Geometry: final body of the model. Coordinates: model frame, mm. A direction names the side the tool comes from. Coordinates: 2 decimals unless noted, no trailing zeros. Loops run counter-clockwise (first coordinate to the right, second up) from the corner with the lowest first, then second, coordinate; pieces in that order, holes last. Notation, with made-up numbers: (47.5, 15) - (86.5, 15) arc R11 cw to (86.5, 36) - close; hole circle Ø10 at (36, 35.5). An arc over 180 degrees is marked (long way). Answer in a Markdown table with one row per item.
from build123d import *

# Parameters (mm, degrees)
BOSS_EXTRUDE1_DEPTH = 8.42
CUT_EXTRUDE1_REACH  = 32.206
SKETCH2_R           = 1.75
SKETCH3_R           = 3
CUT_EXTRUDE2_DEPTH  = 3
CUT_EXTRUDE3_DEPTH  = 3


with BuildPart() as part:
    # Sketch1 → Boss-Extrude1 (new body)
    with BuildSketch(Plane.XY):
        with BuildLine():
            Line((-6.1, -6.416432818), (-6.1, -11.91))
            ThreePointArc((-6.1, -11.91), (-6.246446609, -12.263553391), (-6.6, -12.41))
            Line((-6.6, -12.41), (-12.61, -12.41))
            ThreePointArc((-12.61, -12.41), (-12.963553391, -12.263553391), (-13.11, -11.91))
            Line((-13.11, -11.91), (-13.11, -4.49))
            ThreePointArc((-13.11, -4.49), (-12.963553391, -4.136446609), (-12.61, -3.99))
            Line((-12.61, -3.99), (-10.61, -3.99))
            ThreePointArc((-10.61, -3.99), (-10.256446609, -3.843553391), (-10.11, -3.49))
            Line((-10.11, -3.49), (-10.11, 0))
            ThreePointArc((-10.11, 0), (0, 10.11), (10.11, 0))
            Line((10.11, 0), (10.11, -3.49))
            ThreePointArc((10.11, -3.49), (10.256446609, -3.843553391), (10.61, -3.99))
            Line((10.61, -3.99), (12.61, -3.99))
            ThreePointArc((12.61, -3.99), (12.963553391, -4.136446609), (13.11, -4.49))
            Line((13.11, -4.49), (13.11, -11.91))
            ThreePointArc((13.11, -11.91), (12.963553391, -12.263553391), (12.61, -12.41))
            Line((12.61, -12.41), (6.6, -12.41))
            ThreePointArc((6.6, -12.41), (6.246446609, -12.263553391), (6.1, -11.91))
            Line((6.1, -11.91), (6.1, -6.416432818))
            ThreePointArc((6.1, -6.416432818), (6.037104415, -5.625863403), (5.85, -4.855183318))
            ThreePointArc((5.85, -4.855183318), (5.600165486, -3.334613501), (5.825225225, -1.810179846))
            ThreePointArc((5.825225225, -1.810179846), (0, 6.1), (-5.825225225, -1.810179846))
            ThreePointArc((-5.825225225, -1.810179846), (-5.600165486, -3.334613501), (-5.85, -4.855183318))
            ThreePointArc((-5.85, -4.855183318), (-6.037104415, -5.625863403), (-6.1, -6.416432818))
        make_face()
    extrude(amount=BOSS_EXTRUDE1_DEPTH)

    # Cut-Extrude1: up to this face of the body (flat: up to its plane)
    cut_extrude1_end = Plane(part.part.faces().sort_by_distance((-13.11, -8.2, 4.21))[0])
    # Sketch2 → Cut-Extrude1 (cut, up to the picked face)
    with BuildSketch(Plane(origin=(13.11, 0, 0), x_dir=(0, 0, -1), z_dir=(1, 0, 0)), mode=Mode.PRIVATE) as cut_extrude1_sk1:
        with Locations((-4.21, -8.2)):
            Circle(SKETCH2_R)
    cut_extrude1_tool1 = split(extrude(cut_extrude1_sk1.sketch, amount=-CUT_EXTRUDE1_REACH, mode=Mode.PRIVATE), bisect_by=cut_extrude1_end, keep=Keep.BOTH, mode=Mode.PRIVATE)
    add(cut_extrude1_tool1.solids().sort_by(Axis((13.11, -8.2, 4.21), (-1, 0, 0)))[0], mode=Mode.SUBTRACT)

    # Sketch3 → Cut-Extrude2 (cut)
    with BuildSketch(Plane(origin=(13.11, 0, 0), x_dir=(0, 0, -1), z_dir=(1, 0, 0))):
        with Locations((-4.21, -8.2)):
            Circle(SKETCH3_R)
    extrude(amount=-CUT_EXTRUDE2_DEPTH, mode=Mode.SUBTRACT)

    # Sketch4 → Cut-Extrude3 (cut)
    with BuildSketch(Plane.ZY.offset(13.11)):
        Polygon((7.443161507, -8.2), (5.826580754, -5.4), (2.593419246, -5.4), (0.976838493, -8.2), (2.593419246, -11), (5.826580754, -11), align=None)
    extrude(amount=-CUT_EXTRUDE3_DEPTH, mode=Mode.SUBTRACT)


solid = part.part
(1) Cut plane C-C on x = 0. Output: boundary loops of the cut face in (y, z).
Verdict:
| item | result |
|---|---|
| outline | (6.1, 0) - (10.11, 0) - (10.11, 8.42) - (6.1, 8.42) - close |
(2) Ray query, probe 1 along Y at (x, z) = (-11.25, 3); probe 2 along X at (y, z) = (-3.25, 5); probe 3 along Y at (x, z) = (0, 6.25). Return the intervals inside material, ascending.
Verdict:
| item | result |
|---|---|
| probe 1 | y = -12.41 to -11, -5.4 to -3.99 |
| probe 2 | x = -10.11 to -5.6, 5.6 to 10.11 |
| probe 3 | y = 6.1 to 10.11 |
(3) Access query for faces 4 (the face through (-11.631, -9.62, 6.624)), 5 (the face through (-10.11, -2, 4)), 6 (the face through (10.11, -2, 4)). Directions: +Z, -Z, +X, -X, +Y, -Y. A direction counts if a zero-diameter tool reaches every point of the face in a straight line with its end or side. Return the directions, or none.
Verdict:
| item | result |
|---|---|
| face 4 | -X |
| face 5 | +Z, -Z, -X, +Y |
| face 6 | +Z, -Z, +X, +Y |
(4) Cut plane A-A on x = 7.25. Output: boundary loops of the cut face in (y, z).
Verdict:
| item | result |
|---|---|
| outline | (-12.41, 0) - (7.05, 0) - (7.05, 8.42) - (-12.41, 8.42) - close; hole circle Ø3.5 at (-8.2, 4.21) |
(5) Cut plane D-D on y = 7. Output: boundary loops of the cut face in (x, z).
Verdict:
| item | result |
|---|---|
| outline | (-7.29, 0) - (7.29, 0) - (7.29, 8.42) - (-7.29, 8.42) - close |
(6) First-contact query: pin 1 Ø2.5 at (y, z) = (-8.5, 3) entering from -X; pin 2 Ø1 at (x, z) = (-4.5, 1.5) entering from +Y; pin 3 Ø5 at (x, y) = (-6, -7.5) entering from -Z; pin 4 Ø1.5 at (x, z) = (-11, 4.5) entering from +Y. Flat tips, straight axial feed; report the tip coordinate or a pass-through.
Verdict:
| item | result |
|---|---|
| pin 1 | stops at x = -10.11 |
| pin 2 | stops at y = 9.29 |
| pin 3 | stops at z = 0 |
| pin 4 | stops at y = -3.84 |
(7) Cut plane B-B on z = 4.21. State how many separate pieces and enclosed holes the cut face has, then the cut area to 3 significant figures.
Verdict:
| item | result |
|---|---|
| separate pieces | 3 |
| enclosed holes | 0 |
| area | 192 mm² |
(8) Pull-direction query (X, two-part tool) for faces 1 (the face through (-0.222, 10.108, 4.151)), 2 (the face through (-11.631, -6.78, 1.796)), 3 (the face through (6.1, -10.4, 4.2)); classes: pulls with the +X half, pulls with the -X half, needs draft (parallel to the pull), parting line crosses it, or undercut.
Verdict:
| item | result |
|---|---|
| face 1 | parting line crosses it |
| face 2 | needs draft |
| face 3 | undercut |
